Design review of the part shown in the three views and the two pictorial views. Dimensions are in mm from the part's minimum x, y and z. A direction names the side the tool comes from. Round coordinates to 2 decimals unless told otherwise and drop trailing zeros. Loops run counter-clockwise (first coordinate to the right, second up) from the corner with the lowest first, then second, coordinate; pieces in that order, holes last.
1. Consider section D-D on z = 4.55. State the section outline as (x, y) points, then the cut area to 3 significant figures.
2. Consider section C-C on z = 3. State the section outline as (x, y) points, then the cut area to 3 significant figures.
3. Clearance check with flat-ended pins moving along their axes: pin 1 Ø3 at (x, z) = (6.5, 0.5) entering from +Y; pin 2 Ø2 at (y, z) = (10.5, 3.5) entering from +X. State where each tip first meets the part, or that it passes through.
4. Tool access review of the marked faces 1 and 2: name each direction out of +Z, -Z, +X, -X, +Y, -Y from which nothing blocks a thin tool from reaching the whole face with its end or side.
5. Consider section A-A on x = 15. State the section outline as (y, z) points.
6. To check wall thickness, follow line 1 along Z through (x, y) = (3.75, 22.75); line 2 along Y through (x, z) = (15, 3.55); line 3 along X through (y, z) = (15.25, 4.15). State the ranges of each line that lie inside material, in increasing order.
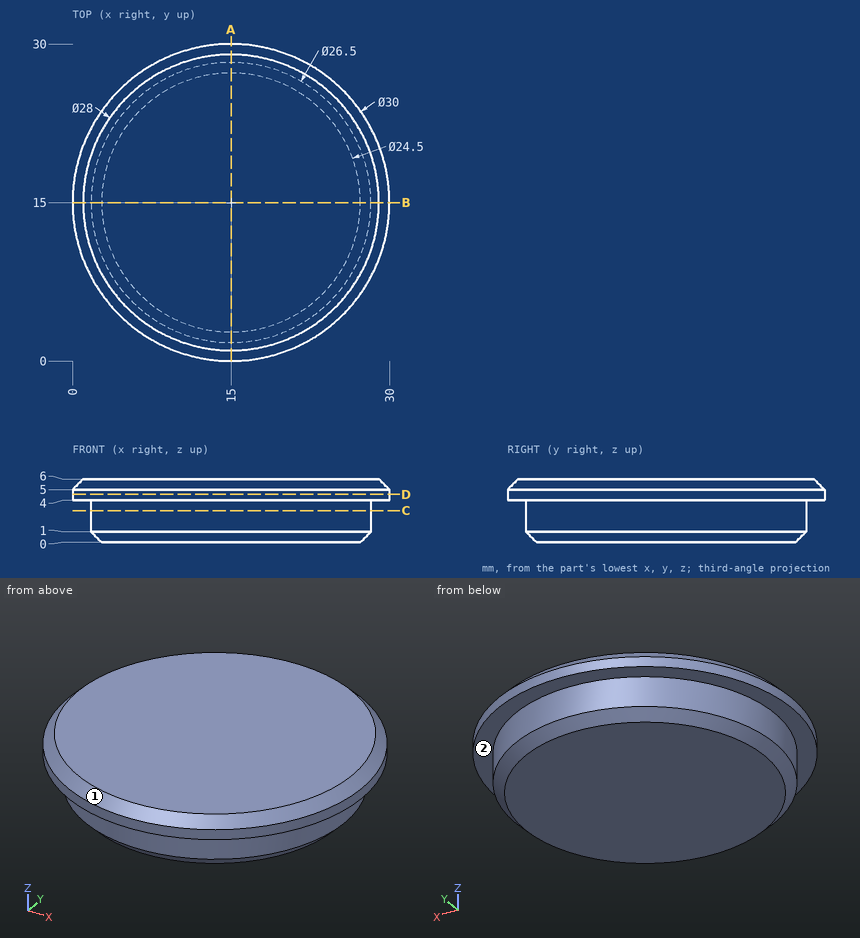
Resolved:
1. outline: circle Ø30 at (15, 15)
1. area: 707 mm2
2. outline: circle Ø26.5 at (15, 15)
2. area: 552 mm2
3. pin 1: stops at y = 26.2
3. pin 2: stops at x = 29.55
4. face 1: +Z
4. face 2: -Z
5. outline: (0, 4) - (1.75, 4) - (1.75, 1) - (2.75, 0) - (27.25, 0) - (28.25, 1) - (28.25, 4) - (30, 4) - (30, 5) - (29, 6) - (1, 6) - (0, 5) - close
6. line 1: z = 4 to 6
6. line 2: y = 1.75 to 28.25
6. line 3: x = 0 to 30
